The listing builds one solid part. Answer for the finished solid, in the listing's coordinates (mm). A direction names the side the tool comes from. Give positions to 0.01 mm unless a question says otherwise; leave off trailing zeros. Loops run counter-clockwise (first coordinate to the right, second up) from the corner with the lowest first, then second, coordinate; pieces in that order, holes last.
Item 1: Each of these flat-tipped pins is pushed along its axis until it touches: pin 1 Ø2 at (x, z) = (15, -0.5) entering from -Y; pin 2 Ø3 at (y, z) = (9, 1) entering from -X; pin 3 Ø2 at (x, z) = (-15, 0) entering from -Y; pin 4 Ø1 at (x, z) = (1, 0) entering from +Y. Where does it stop, or does it pass through?
Item 2: Section B-B, the plane y = 10 is taken. Give the vertices of the cut face in (x, z) (3 decimals), and give its area (3 significant figures).
Item 3: A tool of negligible diameter and unlimited length cuts with its end or side. For faces 5 (the face through (17.5, 1, 0)), 6 (the face through (13.75, 0.99, 0.05)), from which of +Z, -Z, +X, -X, +Y, -Y can it reach the whole face along a straight path? Write none if from no direction.
Item 4: The mould has two halves that part along X. Classify faces 1 (the face through (-16.25, 0.99, 0.05)), 2 (the face through (0, 1, 2.5)), 3 (the face through (-17.5, 1, 0)), 4 (the face through (0.05, 10.99, 0.04)): pulls with the +X half, pulls with the -X half, needs draft (parallel to the pull), parting line crosses it, or undercut.
Item 5: Section A-A, the plane x = -3 is taken. Give the vertices of the cut face in (y, z), and give its area (3 significant figures).
Item 6: Consider line 1 along Z through (x, y) = (15, 1.3); line 2 along Y through (x, z) = (-2.5, 1.65); line 3 along X through (y, z) = (6.5, 0.55). Determine where each line is inside the solid, lowest interval first.
Autodesk Inventor part; units mm, degrees
ref_plane "YZ Plane" through (0, 0, 0) normal (1, 0, 0) x (0, 1, 0)
ref_plane "XZ Plane" through (0, 0, 0) normal (0, 1, 0) x (-1, 0, 0)
ref_plane "XY Plane" through (0, 0, 0) normal (0, 0, 1) x (1, 0, 0)
sketch "Sketch1" plane through (0, 0, 0) normal (0, 1, 0) x (-1, 0, 0)
  line L0 (-17.5, 2.5) -> (17.5, 2.5)
  line L1 (17.5, 2.5) -> (17.5, -2.5)
  line L2 (17.5, -2.5) -> (-17.5, -2.5)
  line L3 (-17.5, -2.5) -> (-17.5, 2.5)
  line L4 (-17.5, 2.5) -> (17.5, -2.5) construction
  line L5 (17.5, 2.5) -> (-17.5, -2.5) construction
  line L6 (-10, 2.5) -> (10, 2.5)
  line L7 (10, 2.5) -> (10, -2.5)
  line L8 (10, -2.5) -> (-10, -2.5)
  line L9 (-10, -2.5) -> (-10, 2.5)
  line L10 (-10, 2.5) -> (10, -2.5) construction
  line L11 (10, 2.5) -> (-10, -2.5) construction
  point P0 (0, 0)
  dimension "d0" = 35
  dimension "d1" = 5
  dimension "d2" = 20
extrude "Extrusion1" add sketch "Sketch1" along normal blind 2.5 contours L0 L9 L2 L3 | L0 L1 L2 L7
extrude "Extrusion2" add sketch "Sketch1" along normal blind 30 contours L0 L7 L2 L9
sketch "Sketch2" plane through (-17.5, 0, 2.5) normal (0, 0, 1) x (1, 0, 0)
  line L0 (0, 2.5) -> (7.5, 2.5)
  line L1 (27.5, 2.5) -> (35, 2.5)
  line L2 (27.5, 2.5) -> (27.5, 30)
  line L3 (7.5, 2.5) -> (7.5, 30)
  line L4 (7.5, 30) -> (27.5, 30)
  line L5 (35, 0) -> (0, 0)
  line L6 (0, 0) -> (0, 2.5)
  line L7 (35, 0) -> (35, 2.5)
  line L8 (7.5, 2.5) -> (0, 2.5)
  line L9 (0, 0) -> (35, 0)
  circle A0 centre (17.4535, 4.99) radius 3.595
  circle A1 centre (17.4535, 4.99) radius 6
  line L10 (12.1387, 7.7745) -> (11.4535, 5.8766) construction
  line L11 (11.4535, 5.8766) -> (8.7602, 4.0511) construction
  line L12 (8.7602, 4.0511) -> (4.3576, 3.0847) construction
  line L13 (4.3576, 3.0847) -> (0, 2.5) construction
  spline S0 degree 4 poles (12.1387, 7.7745) (11.4535, 5.8766) (8.7602, 4.0511) (4.3576, 3.0847) (0, 2.5) knots 1 1 1 1 1 2 2 2 2 2
  line L14 (17.4535, 4.99) -> (17.4535, 2.7924)
  line L15 (22.7682, 7.7745) -> (23.4535, 5.8766) construction
  line L16 (23.4535, 5.8766) -> (26.1467, 4.0511) construction
  line L17 (26.1467, 4.0511) -> (30.5493, 3.0847) construction
  line L18 (30.5493, 3.0847) -> (34.907, 2.5) construction
  spline S1 degree 4 poles (22.7682, 7.7745) (23.4535, 5.8766) (26.1467, 4.0511) (30.5493, 3.0847) (34.907, 2.5) knots 1 1 1 1 1 2 2 2 2 2
  point P0 (17.5, 0)
  point P1 (17.5, 0)
  point P2 (17.5, 0)
  point P3 (17.5, 0)
  point P4 (7.5, 10.9282)
  point P5 (27.5, 10.9282)
  point P6 (17.5, 0)
  point P7 (7.5, 6.3541)
  point P8 (27.5, 4.99)
  point P9 (7.5, 6.3541)
  point P10 (7.5, 4.2058)
  point P11 (11.9072, 7.2788)
  point P12 (22.9998, 7.2788)
  point P13 (27.5, 4.171)
  dimension "d77" = 12
  dimension "d58" = 7.19
  dimension "d59" = 4.99
extrude "Extrusion10" cut sketch "Sketch2" against normal blind 19.9625 contours A0
sketch "Sketch4" plane through (0, 0, 0) normal (0, -1, 0) x (1, 0, 0)
  line L0 (-17.5, -2.5) -> (-17.5, 2.5)
  line L1 (17.5, 2.5) -> (17.5, -2.5)
  circle A0 centre (-15, 0) radius 1.25
  line L2 (0, 0) -> (0, -2.2374)
  circle A1 centre (15, 0) radius 1.25
  point P0 (-17.5, 0)
  point P1 (17.5, 0)
  dimension "d68" = 2.5
  dimension "d71" = 2.5
  dimension "d72" = 2.5
extrude "Extrusion14" cut sketch "Sketch4" against normal blind 2
extrude "Extrusion17" cut sketch "Sketch2" against normal blind 5 contours L3 L4 L2 S1 A1 S0
extrude "Extrusion18" add sketch "Sketch2" against normal blind 5 contours S0 L3 L0 | S1 L1 L2
properties part number "chassis 2"
Worked answers:
1. pin 1: stops at y = 0
1. pin 2: stops at x = -5.5
1. pin 3: stops at y = 2
1. pin 4: stops at y = 10.97
2. outline: (-3.348, -2.5) - (3.255, -2.5) - (3.255, 2.5) - (-3.348, 2.5) - close
2. area: 33.0 mm2
3. face 5: +Z, -Z, +X, +Y, -Y
3. face 6: -Y
4. face 1: undercut
4. face 2: needs draft
4. face 3: pulls with the -X half
4. face 4: parting line crosses it
5. outline: (0, -2.5) - (2.94, -2.5) - (2.94, 2.5) - (0, 2.5) - close; (7.04, -2.5) - (10.21, -2.5) - (10.21, 2.5) - (7.04, 2.5) - close
5. area: 30.6 mm2
6. line 1: z = -2.5 to -1.25, 1.25 to 2.5
6. line 2: y = 0 to 2.36, 7.62 to 10.47
6. line 3: x = -6.18 to -3.31, 3.22 to 6.09
